Build history of the part. All positions in model axes, mm. A direction names the side the tool comes from. Round coordinates to 2 decimals unless told otherwise and drop trailing zeros. Write each loop counter-clockwise with the first axis right and the second up, starting at its lowest first coordinate (ties: lowest second). Pieces come first, ordered by that corner, then holes.
Item 1: 3-axis set-ups, long thin cutter, end or side, ignore diameter. For faces 1 (the flat face through (9, 5, 9)), 2 (the flat face through (8, 5, 3)), 3 (the flat face through (0, 5, 3)): which of +Z, -Z, +X, -X, +Y, -Y reach the whole face in a straight line?
Item 2: Wall check: probe 1 along X at (y, z) = (3.75, 6.5); probe 2 along X at (y, z) = (9.75, 7.75); probe 3 along Z at (x, y) = (-0.25, 4) (3 decimals). Give the ranges that are in metal, low to high.
Item 3: Band-saw the part on A-A, the plane y = 7.5. Write the cut outline in (x, z), then the cut area to 3 significant figures.
Item 4: Band-saw the part on C-C, the plane x = 8.25. Write the cut outline in (y, z) (3 decimals), then the cut area to 4 significant figures.
Item 5: Band-saw the part on B-B, the plane z = 1. Write the cut outline in (x, y).
Item 6: Drop flat-ended pins along their axis: pin 1 Ø2 at (y, z) = (3.5, 2.5) entering from -X; pin 2 Ø1.5 at (y, z) = (6.5, 6.5) entering from -X; pin 3 Ø5.5 at (y, z) = (4.5, 4.5) entering from +X. Give the stop position or say it passes through.
Solid Edge part; units mm, degrees
sketch "Sketch1" plane through (0, 0, 0) normal (0, -1, 0) x (1, 0, 0)
  line L0 (9, 10) -> (-1, 10)
  line L1 (-1, 10) -> (-1, 8.5)
  line L2 (0, 7) -> (-1, 8.5)
  line L3 (0, 0) -> (0, 7)
  line L4 (0, 0) -> (8, 0)
  line L5 (8, 0) -> (8, 7)
  line L6 (9, 8.5) -> (8, 7)
  line L7 (9, 10) -> (9, 8.5)
extrude "Protrusion1" add sketch "Sketch1" against normal blind 10
properties material "Stainless Steel, 420"
Results:
1. face 1: +Z, -Z, +X, +Y, -Y
1. face 2: -Z, +X, +Y, -Y
1. face 3: -Z, -X, +Y, -Y
2. probe 1: x = 0 to 8
2. probe 2: x = -0.5 to 8.5
2. probe 3: z = 7.375 to 10
3. outline: (-1, 8.5) - (0, 7) - (0, 0) - (8, 0) - (8, 7) - (9, 8.5) - (9, 10) - (-1, 10) - close
3. area: 84.5 mm2
4. outline: (0, 7.375) - (10, 7.375) - (10, 10) - (0, 10) - close
4. area: 26.25 mm2
5. outline: (0, 0) - (8, 0) - (8, 10) - (0, 10) - close
6. pin 1: stops at x = 0
6. pin 2: stops at x = -0.17
6. pin 3: stops at x = 8.17
